from build123d import *

# Parameters (mm, degrees)
SKETCH1_W               = 40
SKETCH1_H               = 40
BOSS_EXTRUDE1_DEPTH     = 20
FILLET1_R               = 1
SKETCH2_R               = 6
BOSS_EXTRUDE2_DEPTH     = 1.5
FILLET2_R               = 1
BOSS_EXTRUDE4_START     = 0.9
SKETCH4_R               = 6
BOSS_EXTRUDE4_DEPTH     = 0.9
FILLET3_R               = 1
CUT_EXTRUDE2_DEPTH      = 55.163169457
CUT_EXTRUDE2_DEPTH_BACK = 55.163169457
SKETCH3_R               = 3


with BuildPart() as part:
    # Sketch1 → Boss-Extrude1 (new body)
    with BuildSketch(Plane(origin=(0, 0, 0), x_dir=(0, 0, -1), z_dir=(1, 0, 0))):
        with Locations((6.618181818, -7.127272727)):
            Rectangle(SKETCH1_W, SKETCH1_H)
    extrude(amount=BOSS_EXTRUDE1_DEPTH)

    # Fillet1
    fillet1_edges = [part.edges().sort_by_distance(p)[0] for p in [
        (20, -7.127272727, -26.618181818),
        (20, 12.872727273, -6.618181818),
        (20, -7.127272727, 13.381818182),
        (0, 12.872727273, -6.618181818),
        (0, -7.127272727, -26.618181818),
        (0, -27.127272727, -6.618181818),
        (0, -7.127272727, 13.381818182),
        (20, -27.127272727, -6.618181818),
        (10, 12.872727273, 13.381818182),
        (10, 12.872727273, -26.618181818),
        (10, -27.127272727, -26.618181818),
        (10, -27.127272727, 13.381818182),
    ]]
    fillet(fillet1_edges, radius=FILLET1_R)

    # Sketch2 → Boss-Extrude2 (add)
    with BuildSketch(Plane.XY.offset(13.381818182)):
        with Locations(Location((10, 2.872727273, 0), (0, 0, 180))):
            Circle(SKETCH2_R)
    extrude(amount=BOSS_EXTRUDE2_DEPTH)

    # Fillet2
    fillet2_edges = [part.edges().sort_by_distance(p)[0] for p in [
        (16, 2.872727273, 14.881818182),
    ]]
    fillet(fillet2_edges, radius=FILLET2_R)

    # Sketch4 → Boss-Extrude4 (add)
    with BuildSketch(Plane(origin=(0, 0, -26.618181818), x_dir=(-1, 0, 0), z_dir=(0, 0, -1)).offset(BOSS_EXTRUDE4_START)):
        with Locations((-10, 2.872727273)):
            Circle(SKETCH4_R)
    extrude(amount=-BOSS_EXTRUDE4_DEPTH)

    # Fillet3
    # the kernel refuses this fillet: 1 mm, written as the material it takes off along each edge
    with BuildSketch(Plane(origin=(10, 2.872727273, -27.518181818), x_dir=(-1, 0, 0), z_dir=(0, -1, 0))) as fillet3_piece_1:
        with BuildLine():
            CenterArc((5.005012563, -1), FILLET3_R, 5.739170477, 84.260829523)
            Line((5.005012563, 0), (5.005012563, 0.02))
            Line((5.005012563, 0.02), (6, 0.02))
            Line((6, 0.02), (6.02, 0))
            ThreePointArc((6.02, 0), (6.02, -0.45), (6.019899749, -0.898))
            Line((6.019899749, -0.898), (6, -0.9))
        make_face()
    revolve(axis=Axis((10, 2.872727273, -27.518181818), (0, 0, -1)), mode=Mode.SUBTRACT)

    # Sketch3 → Cut-Extrude2 (cut, two sides: drawn at the far end of the back side and taken through both)
    with BuildSketch(Plane.XY.offset(14.881818182).offset(-CUT_EXTRUDE2_DEPTH_BACK)):
        with Locations(Location((10, 2.872727273, 0), (0, 0, 180))):
            Circle(SKETCH3_R)
    extrude(amount=CUT_EXTRUDE2_DEPTH + CUT_EXTRUDE2_DEPTH_BACK, mode=Mode.SUBTRACT)


solid = part.part
Model file for the job. Use its own axes, mm. A direction names the side the tool comes from. Round coordinates to 2 decimals unless told otherwise and drop trailing zeros. Loops run counter-clockwise (first coordinate to the right, second up) from the corner with the lowest first, then second, coordinate; pieces in that order, holes last. Notation, with made-up numbers: (29.5, 33.5) -> (55.5, 33.5) arc R34 cw to (55.5, 66.5) -> close; hole circle Ø8 at (13, 51.25). An arc over 180 degrees is marked (long way). Answer as CSV lines item,"result". Start each with the question number.
1) Slice it at B-B (x = 10). List the corners of the cut face in (y, z).
2) Slice it at A-A (y = -8). List the corners of the cut face in (x, z), plus the area to 3 significant figures.
3) Probe line 1 along Y through (x, z) = (10, 6.5); line 2 along X through (y, z) = (3, -24); line 3 along Z through (x, y) = (16.5, 0). List the from-to ranges inside material, lowest first.
4) Pin check, flat tips, straight feed: P1, Ø1.5, axis at x = 17.5, y = -13.5, coming from the -Z side; P2, Ø7, axis at x = 10, y = 2.87, coming from the -Z side. Stop position of each tip, or through.
5) Slice it at C-C (z = -19). List the corners of the cut face in (x, y), plus the area to 3 significant figures.
6) Mould opens along Y. For faces 1 (the face through (19.699, 12.588, -6.884)), 2 (the face through (12.38, 4.7, -6.61)), 3 (the face through (19.7, -26.84, -6.88)), 4 (the face through (10, -7, 13.382)) say: +Y half, -Y half, draft (parallel to the pull), parting line (faces both ways), or undercut.
7) Tool access for faces 5 (the face through (19.7, -6.86, -26.33)), 6 (the face through (7.231, 8.196, 13.628)): list every direction of +Z, -Z, +X, -X, +Y, -Y with a clear straight run to the whole face (end or side of a thin tool).
Filled in:
1,outline,"(-27.13, -25.62) arc R1 ccw to (-26.13, -26.62) -> (-3.13, -26.62) arc R1 ccw to (-2.13, -27.52) -> (-0.13, -27.52) -> (-0.13, 14.88) -> (-2.13, 14.88) arc R1 ccw to (-3.13, 13.88) -> (-3.13, 13.38) -> (-26.13, 13.38) arc R1 ccw to (-27.13, 12.38) -> close; (5.87, -27.52) -> (7.88, -27.52) arc R1 ccw to (8.87, -26.62) -> (11.87, -26.62) arc R1 ccw to (12.87, -25.62) -> (12.87, 12.38) arc R1 ccw to (11.87, 13.38) -> (8.87, 13.38) -> (8.87, 13.88) arc R1 ccw to (7.87, 14.88) -> (5.87, 14.88) -> close"
2,outline,"(0, -25.62) arc R1 ccw to (1, -26.62) -> (19, -26.62) arc R1 ccw to (20, -25.62) -> (20, 12.38) arc R1 ccw to (19, 13.38) -> (1, 13.38) arc R1 ccw to (0, 12.38) -> close"
2,area,"799 mm2"
3,line 1,"y = -27.13 to -0.13, 5.87 to 12.87"
3,line 2,"x = 0 to 7, 13 to 20"
3,line 3,"z = -26.62 to 13.38"
4,P1,"stops at z = -26.62"
4,P2,"stops at z = -27.52"
5,outline,"(0, -26.13) arc R1 ccw to (1, -27.13) -> (19, -27.13) arc R1 ccw to (20, -26.13) -> (20, 11.87) arc R1 ccw to (19, 12.87) -> (1, 12.87) arc R1 ccw to (0, 11.87) -> close; hole circle Ø6 at (10, 2.87)"
5,area,"771 mm2"
6,face 1,"+Y half"
6,face 2,"undercut"
6,face 3,"-Y half"
6,face 4,"draft"
7,face 5,"-Z, +X, +Y, -Y"
7,face 6,"+Z"
